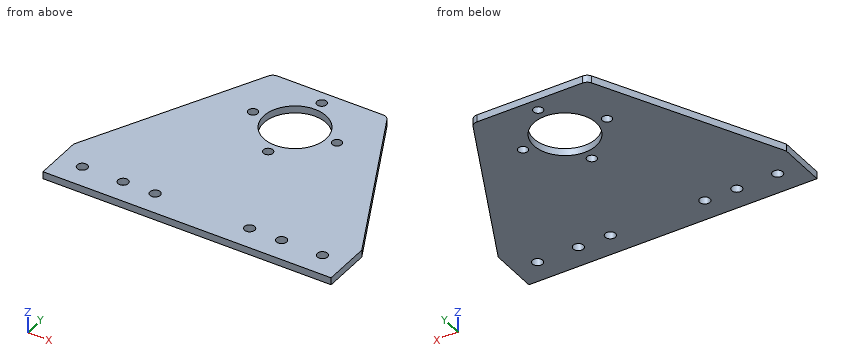
from build123d import *

# Parameters (mm, degrees)
SKETCH1_R      = 2.15
EXTRUDE1_DEPTH = 3


with BuildPart() as part:
    # Sketch1 → Extrude1 (new body)
    with BuildSketch(Plane.XY):
        with BuildLine():
            Line((46.447148798, 50.325025124), (11.138674094, -21.397126503))
            Line((11.138674094, -21.397126503), (11.138674094, -41.397126503))
            Line((11.138674094, -41.397126503), (131.138674094, -41.397126503))
            Line((131.138674094, -41.397126503), (131.138674094, -21.397126503))
            Line((131.138674094, -21.397126503), (95.830199391, 50.325025124))
            ThreePointArc((95.830199391, 50.325025124), (94.723748955, 51.547064523), (93.138674094, 52))
            Line((93.138674094, 52), (49.138674094, 52))
            ThreePointArc((49.138674094, 52), (47.553599234, 51.547064523), (46.447148798, 50.325025124))
        make_face()
        with Locations((21.138674094, -31.397126503)):
            Circle(SKETCH1_R, mode=Mode.SUBTRACT)
        with Locations((121.138674094, -31.397126503)):
            Circle(SKETCH1_R, mode=Mode.SUBTRACT)
        with Locations((104.138674094, -31.397126503)):
            Circle(SKETCH1_R, mode=Mode.SUBTRACT)
        with Locations((90.827251635, -31.397126503)):
            Circle(SKETCH1_R, mode=Mode.SUBTRACT)
        with Locations((51.450096554, -31.397126503)):
            Circle(SKETCH1_R, mode=Mode.SUBTRACT)
        with Locations((38.138674094, -31.397126503)):
            Circle(SKETCH1_R, mode=Mode.SUBTRACT)
        with BuildLine():
            ThreePointArc((69.138674094, 11.502873497), (71.138674094, 9.502873497), (73.138674094, 11.502873497))
            ThreePointArc((73.138674094, 11.502873497), (71.138674094, 13.502873497), (69.138674094, 11.502873497))
        make_face(mode=Mode.SUBTRACT)
        with BuildLine():
            ThreePointArc((51.638674094, 29.002873497), (53.638674094, 27.002873497), (55.638674094, 29.002873497))
            ThreePointArc((55.638674094, 29.002873497), (53.638674094, 31.002873497), (51.638674094, 29.002873497))
        make_face(mode=Mode.SUBTRACT)
        with BuildLine():
            ThreePointArc((69.138674094, 46.502873497), (71.138674094, 44.502873497), (73.138674094, 46.502873497))
            ThreePointArc((73.138674094, 46.502873497), (71.138674094, 48.502873497), (69.138674094, 46.502873497))
        make_face(mode=Mode.SUBTRACT)
        with BuildLine():
            ThreePointArc((86.638674094, 29.002873497), (88.638674094, 27.002873497), (90.638674094, 29.002873497))
            ThreePointArc((90.638674094, 29.002873497), (88.638674094, 31.002873497), (86.638674094, 29.002873497))
        make_face(mode=Mode.SUBTRACT)
        with BuildLine():
            ThreePointArc((58.138674094, 29.002873497), (71.138674094, 16.002873497), (84.138674094, 29.002873497))
            ThreePointArc((84.138674094, 29.002873497), (71.138674094, 42.002873497), (58.138674094, 29.002873497))
        make_face(mode=Mode.SUBTRACT)
    extrude(amount=EXTRUDE1_DEPTH)


solid = part.part
The model under review builds one solid part; all positions refer to its coordinate system, in mm. Give positions to 0.01 mm unless a question says otherwise; leave off trailing zeros. Loops run counter-clockwise (first coordinate to the right, second up) from the corner with the lowest first, then second, coordinate; pieces in that order, holes last. Notation, with made-up numbers: (-1.5, 34) -> (17.5, 34) arc R19 ccw to (17.5, 61) -> close; hole circle Ø6 at (24, -21.75). An arc over 180 degrees is marked (long way). Answer as a JSON object with one key per item and string values. Group by question number.
Q1. Take a section at C-C (x = 29). Write out the cut boundary in (y, z).
Q2. Take a section at B-B (z = 1.3). State how many separate pieces and enclosed holes the cut face has, plus the area to 3 significant figures.
Q3. Take a section at A-A (y = 36.5). Write out the cut boundary in (x, z), plus the area to 3 significant figures.
Q4. Take a section at D-D (y = -14). Write out the cut boundary in (x, z).
Q5. Insertion check: pin 1 (3 mm diameter, centred on x = 71.14, y = 46.5, fed in from -Z). The pin has a flat end and moves straight along its axis. Give the tip position at first contact, or say it passes through.
Q6. Wall thickness on line 1 along Y through (x, z) = (70.5, 2.75); line 2 along Y through (x, z) = (70, 2.15); line 3 along X through (y, z) = (22.5, 0.3): over which ranges is each line inside the solid? List them lowest first.
Answer below:
{
 "1": {"outline": "(-41.4, 0) -> (14.88, 0) -> (14.88, 3) -> (-41.4, 3) -> close"},
 "2": {"separate pieces": "1", "enclosed holes": "11", "area": "7,890 mm2"},
 "3": {"outline": "(39.64, 0) -> (60.52, 0) -> (60.52, 3) -> (39.64, 3) -> close; (81.76, 0) -> (102.64, 0) -> (102.64, 3) -> (81.76, 3) -> close", "area": "125 mm2"},
 "4": {"outline": "(14.78, 0) -> (127.5, 0) -> (127.5, 3) -> (14.78, 3) -> close"},
 "5": {"pin 1": "passes through"},
 "6": {"line 1": "y = -41.4 to 9.61, 13.4 to 16.02, 41.99 to 44.61, 48.4 to 52", "line 2": "y = -41.4 to 9.86, 13.15 to 16.05, 41.95 to 44.86, 48.15 to 52", "line 3": "x = 32.75 to 59.88, 82.4 to 109.53"}
}
